The listing builds one solid part. Answer for the finished solid, in the listing's coordinates (mm). A direction names the side the tool comes from. Round coordinates to 2 decimals unless told otherwise and drop trailing zeros. One line per question, with ' | ' between items. Start each with the question number.
Autodesk Inventor part; units mm, degrees
ref_plane "YZ Plane" through (0, 0, 0) normal (1, 0, 0) x (0, 1, 0)
ref_plane "XZ Plane" through (0, 0, 0) normal (0, 1, 0) x (-1, 0, 0)
ref_plane "XY Plane" through (0, 0, 0) normal (0, 0, 1) x (1, 0, 0)
sketch "스케치1" plane through (0, 0, 0) normal (0, 1, 0) x (-1, 0, 0)
  circle A0 centre (-26.5671, -74.7948) radius 2.15
  circle A1 centre (-19.5671, -81.7948) radius 2
  circle A2 centre (-19.5671, -67.7948) radius 2
  circle A3 centre (-33.5671, -67.7948) radius 2
  circle A4 centre (-33.5671, -81.7948) radius 2
  arc A5 (-29.2171, -65.0948) -> (-29.5171, -64.7948) centre (-29.5171, -65.0948) ccw
  line L0 (-29.5171, -64.7948) -> (-36.2671, -64.7948)
  arc A6 (-36.2671, -64.7948) -> (-36.5671, -65.0948) centre (-36.2671, -65.0948) ccw
  line L1 (-36.5671, -65.0948) -> (-36.5671, -71.8448)
  arc A7 (-36.5671, -71.8448) -> (-36.2671, -72.1448) centre (-36.2671, -71.8448) ccw
  line L2 (-36.2671, -72.1448) -> (-35.0671, -72.1448)
  line L3 (-35.0671, -72.1448) -> (-35.0671, -70.6448)
  line L4 (-35.0671, -70.6448) -> (-31.5671, -70.6448)
  arc A8 (-31.5671, -78.9448) -> (-31.5671, -70.6448) centre (-36.8271, -74.7948) ccw
  line L5 (-31.5671, -78.9448) -> (-35.0671, -78.9448)
  line L6 (-35.0671, -78.9448) -> (-35.0671, -77.4448)
  line L7 (-35.0671, -77.4448) -> (-36.2671, -77.4448)
  arc A9 (-36.2671, -77.4448) -> (-36.5671, -77.7448) centre (-36.2671, -77.7448) ccw
  line L8 (-36.5671, -77.7448) -> (-36.5671, -84.4948)
  arc A10 (-36.5671, -84.4948) -> (-36.2671, -84.7948) centre (-36.2671, -84.4948) ccw
  line L9 (-36.2671, -84.7948) -> (-29.5171, -84.7948)
  arc A11 (-29.5171, -84.7948) -> (-29.2171, -84.4948) centre (-29.5171, -84.4948) ccw
  line L10 (-29.2171, -84.4948) -> (-29.2171, -83.2948)
  line L11 (-29.2171, -83.2948) -> (-30.7171, -83.2948)
  line L12 (-30.7171, -83.2948) -> (-30.7171, -79.7948)
  arc A12 (-22.4171, -79.7948) -> (-30.7171, -79.7948) centre (-26.5671, -85.0548) ccw
  line L13 (-22.4171, -79.7948) -> (-22.4171, -83.2948)
  line L14 (-22.4171, -83.2948) -> (-23.9171, -83.2948)
  line L15 (-23.9171, -83.2948) -> (-23.9171, -84.4948)
  arc A13 (-23.9171, -84.4948) -> (-23.6171, -84.7948) centre (-23.6171, -84.4948) ccw
  line L16 (-23.6171, -84.7948) -> (-16.8671, -84.7948)
  arc A14 (-16.8671, -84.7948) -> (-16.5671, -84.4948) centre (-16.8671, -84.4948) ccw
  line L17 (-16.5671, -84.4948) -> (-16.5671, -77.7448)
  arc A15 (-16.5671, -77.7448) -> (-16.8671, -77.4448) centre (-16.8671, -77.7448) ccw
  line L18 (-16.8671, -77.4448) -> (-18.0671, -77.4448)
  line L19 (-18.0671, -77.4448) -> (-18.0671, -78.9448)
  line L20 (-18.0671, -78.9448) -> (-21.5671, -78.9448)
  arc A16 (-21.5671, -70.6448) -> (-21.5671, -78.9448) centre (-16.3071, -74.7948) ccw
  line L21 (-21.5671, -70.6448) -> (-18.0671, -70.6448)
  line L22 (-18.0671, -70.6448) -> (-18.0671, -72.1448)
  line L23 (-18.0671, -72.1448) -> (-16.8671, -72.1448)
  arc A17 (-16.8671, -72.1448) -> (-16.5671, -71.8448) centre (-16.8671, -71.8448) ccw
  line L24 (-16.5671, -71.8448) -> (-16.5671, -65.0948)
  arc A18 (-16.5671, -65.0948) -> (-16.8671, -64.7948) centre (-16.8671, -65.0948) ccw
  line L25 (-16.8671, -64.7948) -> (-23.6171, -64.7948)
  arc A19 (-23.6171, -64.7948) -> (-23.9171, -65.0948) centre (-23.6171, -65.0948) ccw
  line L26 (-23.9171, -65.0948) -> (-23.9171, -66.2948)
  line L27 (-23.9171, -66.2948) -> (-22.4171, -66.2948)
  line L28 (-22.4171, -66.2948) -> (-22.4171, -69.7948)
  arc A20 (-30.7171, -69.7948) -> (-22.4171, -69.7948) centre (-26.5671, -64.5348) ccw
  line L29 (-30.7171, -69.7948) -> (-30.7171, -66.2948)
  line L30 (-30.7171, -66.2948) -> (-29.2171, -66.2948)
  line L31 (-29.2171, -66.2948) -> (-29.2171, -65.0948)
  circle A21 centre (0, 0) radius 2.15
  circle A22 centre (7, -7) radius 2
  circle A23 centre (7, 7) radius 2
  circle A24 centre (-7, 7) radius 2
  circle A25 centre (-7, -7) radius 2
  arc A26 (-2.65, 9.7) -> (-2.95, 10) centre (-2.95, 9.7) ccw
  line L32 (-2.95, 10) -> (-9.7, 10)
  arc A27 (-9.7, 10) -> (-10, 9.7) centre (-9.7, 9.7) ccw
  line L33 (-10, 9.7) -> (-10, 2.95)
  arc A28 (-10, 2.95) -> (-9.7, 2.65) centre (-9.7, 2.95) ccw
  line L34 (-9.7, 2.65) -> (-8.5, 2.65)
  line L35 (-8.5, 2.65) -> (-8.5, 4.15)
  line L36 (-8.5, 4.15) -> (-5, 4.15)
  arc A29 (-5, -4.15) -> (-5, 4.15) centre (-10.26, 0) ccw
  line L37 (-5, -4.15) -> (-8.5, -4.15)
  line L38 (-8.5, -4.15) -> (-8.5, -2.65)
  line L39 (-8.5, -2.65) -> (-9.7, -2.65)
  arc A30 (-9.7, -2.65) -> (-10, -2.95) centre (-9.7, -2.95) ccw
  line L40 (-10, -2.95) -> (-10, -9.7)
  arc A31 (-10, -9.7) -> (-9.7, -10) centre (-9.7, -9.7) ccw
  line L41 (-9.7, -10) -> (-2.95, -10)
  arc A32 (-2.95, -10) -> (-2.65, -9.7) centre (-2.95, -9.7) ccw
  line L42 (-2.65, -9.7) -> (-2.65, -8.5)
  line L43 (-2.65, -8.5) -> (-4.15, -8.5)
  line L44 (-4.15, -8.5) -> (-4.15, -5)
  arc A33 (4.15, -5) -> (-4.15, -5) centre (0, -10.26) ccw
  line L45 (4.15, -5) -> (4.15, -8.5)
  line L46 (4.15, -8.5) -> (2.65, -8.5)
  line L47 (2.65, -8.5) -> (2.65, -9.7)
  arc A34 (2.65, -9.7) -> (2.95, -10) centre (2.95, -9.7) ccw
  line L48 (2.95, -10) -> (9.7, -10)
  arc A35 (9.7, -10) -> (10, -9.7) centre (9.7, -9.7) ccw
  line L49 (10, -9.7) -> (10, -2.95)
  arc A36 (10, -2.95) -> (9.7, -2.65) centre (9.7, -2.95) ccw
  line L50 (9.7, -2.65) -> (8.5, -2.65)
  line L51 (8.5, -2.65) -> (8.5, -4.15)
  line L52 (8.5, -4.15) -> (5, -4.15)
  arc A37 (5, 4.15) -> (5, -4.15) centre (10.26, 0) ccw
  line L53 (5, 4.15) -> (8.5, 4.15)
  line L54 (8.5, 4.15) -> (8.5, 2.65)
  line L55 (8.5, 2.65) -> (9.7, 2.65)
  arc A38 (9.7, 2.65) -> (10, 2.95) centre (9.7, 2.95) ccw
  line L56 (10, 2.95) -> (10, 9.7)
  arc A39 (10, 9.7) -> (9.7, 10) centre (9.7, 9.7) ccw
  line L57 (9.7, 10) -> (2.95, 10)
  arc A40 (2.95, 10) -> (2.65, 9.7) centre (2.95, 9.7) ccw
  line L58 (2.65, 9.7) -> (2.65, 8.5)
  line L59 (2.65, 8.5) -> (4.15, 8.5)
  line L60 (4.15, 8.5) -> (4.15, 5)
  arc A41 (-4.15, 5) -> (4.15, 5) centre (0, 10.26) ccw
  line L61 (-4.15, 5) -> (-4.15, 8.5)
  line L62 (-4.15, 8.5) -> (-2.65, 8.5)
  line L63 (-2.65, 8.5) -> (-2.65, 9.7)
extrude "돌출1" add sketch "스케치1" along normal blind 500 contours L63 L62 L61 A41 L60 L59 L58 A40 L57 A39 L56 A38 L55 L54 L53 A37 L52 L51 L50 A36 L49 A35 L48 A34 L47 L46 L45 A33 L44 L43 L42 A32 L41 A31 L40 A30 L39 L38 L37 A29 L36 L35 L34 A28 L33 A27 L32 A26
properties part number "Propile_202050" material "알루미늄 6061"
(1) Find section A-A on y = 344. Count the separate pieces of the cut face and the enclosed holes in it, plus the area to 3 significant figures.
(2) A tool of negligible diameter and unlimited length cuts with its end or side. For faces 1 (the cylindrical face through (3.56, 246.5, 0.06)), 2 (the flat face through (2.4, 500, 0.1)), from which of +Z, -Z, +X, -X, +Y, -Y can it reach the whole face along a straight path? Write none if from no direction.
(3) This flat-tipped pin is pushed along its axis until it touches: P1, Ø2.5, axis at x = 0, z = 0, coming from the +Y side. Where does it stop, or does it pass through?
(4) Determine the mould class of faces 3 (the flat face through (2.4, 0, 0.1)), 4 (the cylindrical face through (-0.06, 246.5, 3.56)) for opening direction X: pulls with the +X half, pulls with the -X half, needs draft (parallel to the pull), parting line crosses it, or undercut.
(5) Consider L1, parallel to Z at x = 7, y = 254.5; L2, parallel to Z at x = 0, y = 238; L3, parallel to Z at x = -3.25, y = 427. Determine where each line is inside the solid, lowest interval first.
Answer below:
1) separate pieces: 1 | enclosed holes: 5 | area: 154 mm2
2) face 1: +Y, -Y | face 2: +Z, -Z, +X, -X, +Y
3) P1: through
4) face 3: needs draft | face 4: undercut
5) L1: -10 to -9, -5 to -4.15, 4.15 to 5, 9 to 10 | L2: -3.56 to -2.15, 2.15 to 3.56 | L3: -10 to -8.5, -4.4 to 4.4, 8.5 to 10
